Build history of the part. All positions in model axes, mm. Give positions to 0.01 mm unless a question says otherwise; leave off trailing zeros. Write each loop counter-clockwise with the first axis right and the second up, starting at its lowest first coordinate (ties: lowest second). Pieces come first, ordered by that corner, then holes. Notation, with made-up numbers: (12, -1.75) -> (57, -1.75) arc R27 cw to (57, 22.25) -> close; hole circle Ø5 at (62, 7). An arc over 180 degrees is marked (long way). Put each result on its own line as item: value.
from build123d import *

# Parameters (mm, degrees)
BOSS_EXTRUDE1_DEPTH            = 3.175
M4_CLEARANCE_HOLE1_D           = 4.5
M4_CLEARANCE_HOLE1_CSINK_D     = 4.55
M4_CLEARANCE_HOLE1_CSINK_ANGLE = 90
M8_CLEARANCE_HOLE1_AT_2_COUNT  = 2
M8_CLEARANCE_HOLE1_AT_2_PITCH  = 84
SKETCH9_R                      = 21.275
CENTER_HOLE_DEPTH              = 96.302901976


with BuildPart() as part:
    # Sketch1 → Boss-Extrude1 (new body)
    with BuildSketch(Plane.XY):
        Polygon((-76.2, 54.61), (-76.2, 44.45), (-76.2, -44.45), (76.2, -44.45), (76.2, 44.45), (76.2, 57.15), align=None)
    extrude(amount=BOSS_EXTRUDE1_DEPTH)

    # M4 Clearance Hole1 (through all)
    with Locations(Plane.XY.offset(3.175)):
        with Locations((-69.85, 19.05), (-59.055, 38.1), (0, 38.1), (59.055, 38.1), (69.85, 19.05), (69.85, -19.05), (59.055, -38.1), (0, -38.1), (-59.055, -38.1), (-69.85, -19.05)):
            CounterSinkHole(M4_CLEARANCE_HOLE1_D / 2, M4_CLEARANCE_HOLE1_CSINK_D / 2, counter_sink_angle=M4_CLEARANCE_HOLE1_CSINK_ANGLE)

    # Sketch11 → M8 Clearance Hole1 (revolve, cut)
    with BuildSketch(Plane(origin=(-42, 0, 3.175), x_dir=(0, -1, 0), z_dir=(1, 0, 0))):
        Polygon((0, 0), (0, 3.175), (4.5, 3.175), (4.5, 0.025), (4.525, 0), align=None)
    m8_clearance_hole1 = revolve(axis=Axis((-42, 0, 9.525), (0, 0, -1)), mode=Mode.SUBTRACT)

    # M8 Clearance Hole1 at 2: M8 Clearance Hole1 ×2
    with Locations(*[(i * M8_CLEARANCE_HOLE1_AT_2_PITCH, 0, 0) for i in range(1, M8_CLEARANCE_HOLE1_AT_2_COUNT)]):
        add(m8_clearance_hole1, mode=Mode.SUBTRACT)

    # Sketch9 → Center Hole (cut, through all)
    with BuildSketch(Plane.XY.offset(3.175)):
        Circle(SKETCH9_R)
    extrude(amount=-CENTER_HOLE_DEPTH, mode=Mode.SUBTRACT)


solid = part.part
1) Wall check: L1, parallel to X at y = -38.1, z = 0.9 (3 decimals); L2, parallel to X at y = -19.05, z = 2.4; L3, parallel to Y at x = -58, z = 1.1. Give the ranges that are in metal, low to high.
Filled sheet:
L1: -76.2 to -61.305, -56.805 to -2.25, 2.25 to 56.805, 61.305 to 76.2
L2: -76.2 to -72.1, -67.6 to -9.47, 9.47 to 67.6, 72.1 to 76.2
L3: -44.45 to -40.09, -36.11 to 36.11, 40.09 to 54.91
2) Slice it at C-C (y = -6.5). Write the cut outline in (x, z) (3 decimals), plus the area to 3 significant figures.
Filled sheet:
outline: (-76.2, 0) -> (-20.258, 0) -> (-20.258, 3.175) -> (-76.2, 3.175) -> close; (20.258, 0) -> (76.2, 0) -> (76.2, 3.175) -> (20.258, 3.175) -> close
area: 355 mm2
3) Pull direction Y, two halves, no side cores. Call faces 1 (the flat face through (76.2, 6, 2)), 2 (the cylindrical face through (-16.88, -12.95, 1.61)), 3 (the flat face through (-1, -44.45, 2)), 4 (the cylindrical face through (72.1, 19.1, 1.6)): released by +Y, released by -Y, zero draft, split by the parting line, or undercut.
Filled sheet:
face 1: zero draft
face 2: undercut
face 3: released by -Y
face 4: undercut
4) Slice it at D-D (x = -42). Write the cut outline in (y, z) (3 decimals), plus the area to 3 significant figures.
Filled sheet:
outline: (-44.45, 0) -> (-4.5, 0) -> (-4.5, 3.15) -> (-4.525, 3.175) -> (-44.45, 3.175) -> close; (4.5, 0) -> (55.18, 0) -> (55.18, 3.175) -> (4.525, 3.175) -> (4.5, 3.15) -> close
area: 288 mm2
5) Slice it at A-A (x = 42). Write the cut outline in (y, z) (3 decimals), plus the area to 3 significant figures.
Filled sheet:
outline: (-44.45, 0) -> (-4.5, 0) -> (-4.5, 3.15) -> (-4.525, 3.175) -> (-44.45, 3.175) -> close; (4.5, 0) -> (56.58, 0) -> (56.58, 3.175) -> (4.525, 3.175) -> (4.5, 3.15) -> close
area: 292 mm2
6) Slice it at B-B (y = 38.1). Write the cut outline in (x, z) (3 decimals).
Filled sheet:
outline: (-76.2, 0) -> (-61.305, 0) -> (-61.305, 3.15) -> (-61.33, 3.175) -> (-76.2, 3.175) -> close; (-56.805, 0) -> (-2.25, 0) -> (-2.25, 3.15) -> (-2.275, 3.175) -> (-56.78, 3.175) -> (-56.805, 3.15) -> close; (2.25, 0) -> (56.805, 0) -> (56.805, 3.15) -> (56.78, 3.175) -> (2.275, 3.175) -> (2.25, 3.15) -> close; (61.305, 0) -> (76.2, 0) -> (76.2, 3.175) -> (61.33, 3.175) -> (61.305, 3.15) -> close
